Input: part model. Units: mm. Frame: model coordinates. A direction names the side the tool comes from. Give positions to 0.01 mm unless a question says otherwise; leave off trailing zeros. Order: outer loops, then holes, each group sorted by start corner. A loop starts at its lowest first (then second) coordinate and runs counter-clockwise, first axis right, second up. Notation, with made-up numbers: M -34,69.25 L -3,69.25 A25 cw -3,108.25 Z; hole C 8.5,79.25 d1. An arc over 180 degrees is marked long. Use a Markdown table: item, result.
from build123d import *

# Parameters (mm, degrees)
BOSS_EXTRUDE3_DEPTH  = 99.5
SKETCH1_10_OUTSIDE_W = 1698.732
SKETCH1_10_OUTSIDE_H = 798.732
CUT_EXTRUDE2_DEPTH   = 990.242513239


with BuildPart() as part:
    # Sketch1 → Boss-Extrude3 (new body)
    with BuildSketch(Plane.XY):
        Polygon((-499.5, 399.5), (899.5, 399.5), (899.5, 300), (400, -99.5), (0, -99.5), (-499.5, 300), align=None)
    extrude(amount=BOSS_EXTRUDE3_DEPTH)

    # Sketch1<10> outside → Cut-Extrude2 (cut, through all)
    # profile 1 of 2: a face of its own
    with BuildSketch(Plane.XY):
        with Locations((200, 150)):
            Rectangle(SKETCH1_10_OUTSIDE_W, SKETCH1_10_OUTSIDE_H)
        Polygon((-499.5, 399.5), (899.5, 399.5), (899.5, 300), (400, -99.5), (0, -99.5), (-499.5, 300), align=None, mode=Mode.SUBTRACT)
    # profile 2 of 2: a face of its own
    with BuildSketch(Plane.XY):
        Polygon((0, 0), (400, 0), (800, 300), (-400, 300), align=None)
    extrude(amount=CUT_EXTRUDE2_DEPTH, mode=Mode.SUBTRACT)


solid = part.part
1) Cut plane C-C on y = 233.5. Return loops of the section in (x, z), and give its area (3 significant figures).
Response values:
| item | result |
|---|---|
| outline | M -416.35,0 L -311.33,0 L -311.33,99.5 L -416.35,99.5 Z; M 711.33,0 L 816.35,0 L 816.35,99.5 L 711.33,99.5 Z |
| area | 20,900 mm² |
2) Cut plane B-B on z = 21. Return loops of the section in (x, y), and give its area (3 significant figures).
Response values:
| item | result |
|---|---|
| outline | M -499.5,300 L 0,-99.5 L 400,-99.5 L 899.5,300 L 899.5,399.5 L -499.5,399.5 Z; hole M -400,300 L 0,0 L 400,0 L 800,300 Z |
| area | 259,000 mm² |
3) Material intervals for line 1 (Y direction, x = 247, z = 47.5); line 2 (Y direction, x = 763, z = 45); line 3 (X direction, y = 16.5, z = 90.5), sorted ascending. Write a range as from..to.
Response values:
| item | result |
|---|---|
| line 1 | y = -99.5..0, 300..399.5 |
| line 2 | y = 190.83..272.25, 300..399.5 |
| line 3 | x = -145.04..-22, 422..545.04 |
4) Cut plane D-D on y = -53. Return loops of the section in (x, z).
Response values:
| item | result |
|---|---|
| outline | M -58.14,0 L 458.14,0 L 458.14,99.5 L -58.14,99.5 Z |
5) First-contact query: pin 1 Ø4 at (y, z) = (91, 60) entering from -X; pin 2 Ø3 at (x, z) = (629, 88) entering from -Y. Flat tips, straight axial feed; report the tip coordinate or a pass-through.
Response values:
| item | result |
|---|---|
| pin 1 | stops at x = -240.69 |
| pin 2 | stops at y = 82.45 |
6) Cut plane A-A on x = 229. Return loops of the section in (y, z), and give its area (3 significant figures).
Response values:
| item | result |
|---|---|
| outline | M -99.5,0 L 0,0 L 0,99.5 L -99.5,99.5 Z; M 300,0 L 399.5,0 L 399.5,99.5 L 300,99.5 Z |
| area | 19,800 mm² |
7) Mould query, pull axis X, two halves, no side actions, for faces 3 (the face through (-202.8, 152.1, 49.1)), 4 (the face through (-246.25, 97.45, 49.05)), 5 (the face through (899.5, 350, 49)), 6 (the face through (197, 0, 49)). Classes: released by +X, released by -X, zero draft, split by the parting line, or undercut.
Response values:
| item | result |
|---|---|
| face 3 | undercut |
| face 4 | released by -X |
| face 5 | released by +X |
| face 6 | undercut |
8) Reachability of faces 1 (the face through (-499.5, 349, 49)), 2 (the face through (597.2, 147.9, 49.1)) from +Z, -Z, +X, -X, +Y, -Y: full face, straight path, thin tool, end or side. Return the list, or none.
Response values:
| item | result |
|---|---|
| face 1 | +Z, -Z, -X, +Y, -Y |
| face 2 | +Z, -Z |
